Geometry check sheet. Reference: drawing and pictorial views, mm from the part's lowest x, y, z. A direction names the side the tool comes from. Coordinates: 2 decimals unless noted, no trailing zeros. Loops run counter-clockwise (first coordinate to the right, second up) from the corner with the lowest first, then second, coordinate; pieces in that order, holes last. Notation, with made-up numbers: (1.25, -16.5) - (60.25, -16.5) arc R14 ccw to (60.25, -7.5) - close; hole circle Ø10 at (-6, -23). An arc over 180 degrees is marked (long way). Use a Markdown table: item, result. Add a question column.
1) Go/stop test with flat-tipped pins: P1, Ø5, axis at x = 3.5, y = 8, coming from the +Z side; P2, Ø1, axis at y = 19.5, z = 1.5, coming from the -X side; P3, Ø1, axis at y = 3.5, z = 2, coming from the -X side. Record where each tip stops, or that it passes through.
2) Thickness scan on line 1 (Y direction, x = 11, z = 0.1); line 2 (Y direction, x = 11, z = 2.25); line 3 (Y direction, x = 13.5, z = 5). Record the ranges inside material, lowest first.
3) Tool access check on the marked faces 4, 5 and 6. Record the directions out of +Z, -Z, +X, -X, +Y, -Y that give a thin tool (end or side, any length) a straight path to the whole face; none if there is none.
4) Sectioned sample at A-A, the plane y = 11. Enter the section's corners in (x, z).
5) Draft check along Y on the marked faces 1, 2 and 3. Enter one of: pulls with the +Y half, pulls with the -Y half, needs draft (parallel to the pull), parting line crosses it, or undercut.
6) Sectioned sample at D-D, the plane y = 4.25. Enter the section's corners in (x, z).
7) Sectioned sample at C-C, the plane z = 3.75. Enter the section's corners in (x, y).
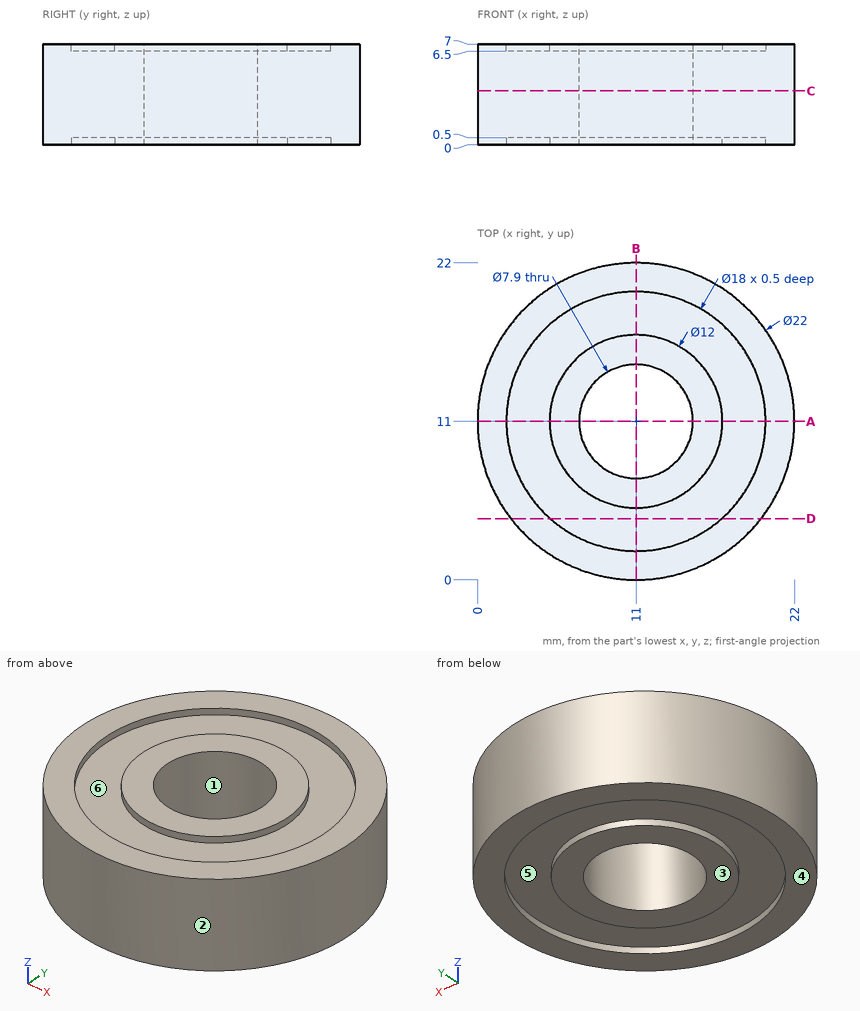
Solved:
| question | item | result |
|---|---|---|
| 1 | P1 | stops at z = 7 |
| 1 | P2 | stops at x = 3.45 |
| 1 | P3 | stops at x = 2.51 |
| 2 | line 1 | y = 0 to 2, 5 to 7.05, 14.95 to 17, 20 to 22 |
| 2 | line 2 | y = 0 to 7.05, 14.95 to 22 |
| 2 | line 3 | y = 0.29 to 7.94, 14.06 to 21.71 |
| 3 | face 4 | -Z, +X, -X, +Y, -Y |
| 3 | face 5 | -Z |
| 3 | face 6 | +Z |
| 4 | outline | (0, 0) - (2, 0) - (2, 0.5) - (5, 0.5) - (5, 0) - (7.05, 0) - (7.05, 7) - (5, 7) - (5, 6.5) - (2, 6.5) - (2, 7) - (0, 7) - close; (14.95, 0) - (17, 0) - (17, 0.5) - (20, 0.5) - (20, 0) - (22, 0) - (22, 7) - (20, 7) - (20, 6.5) - (17, 6.5) - (17, 7) - (14.95, 7) - close |
| 5 | face 1 | undercut |
| 5 | face 2 | parting line crosses it |
| 5 | face 3 | needs draft |
| 6 | outline | (2.31, 0) - (5.05, 0) - (5.05, 0.5) - (16.95, 0.5) - (16.95, 0) - (19.69, 0) - (19.69, 7) - (16.95, 7) - (16.95, 6.5) - (5.05, 6.5) - (5.05, 7) - (2.31, 7) - close |
| 7 | outline | circle Ø22 at (11, 11); hole circle Ø7.9 at (11, 11) |
